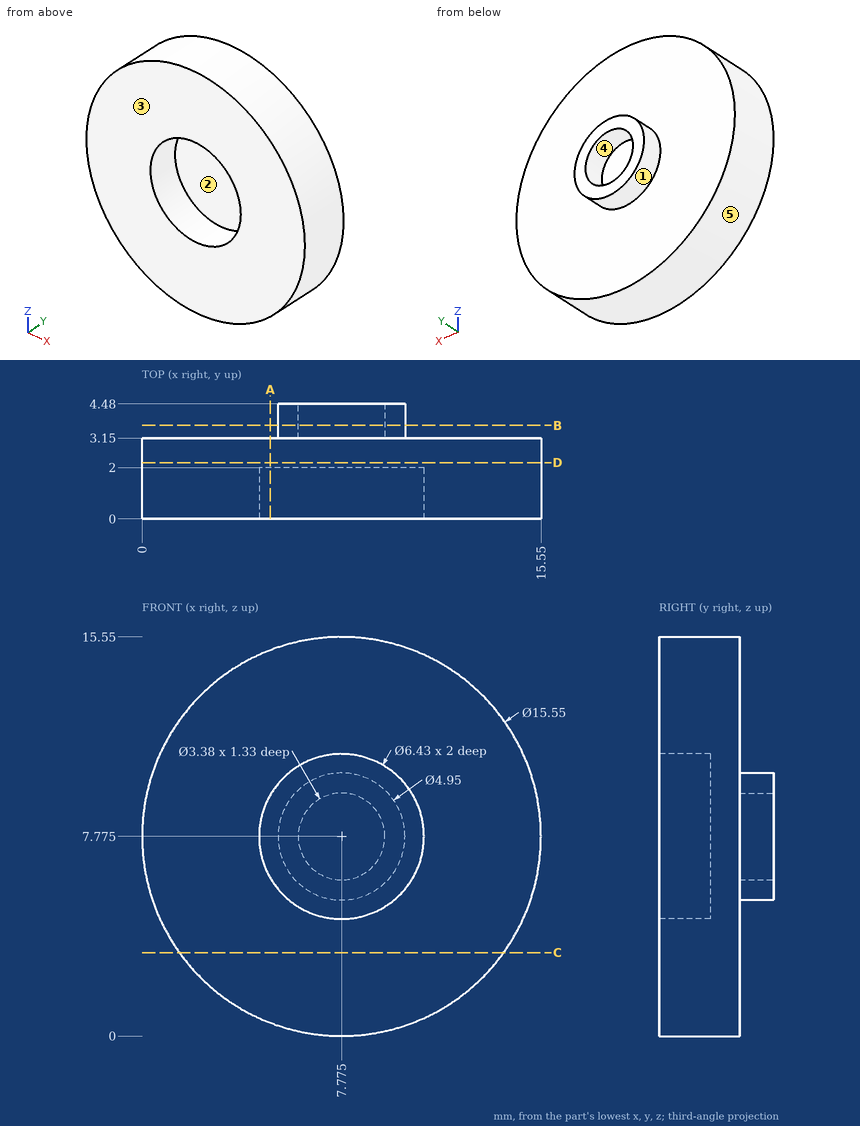
Geometry check sheet. Reference: drawing and pictorial views, mm from the part's lowest x, y, z. A direction names the side the tool comes from. Coordinates: 2 decimals unless noted, no trailing zeros. Order: outer loops, then holes, each group sorted by start corner. A loop starts at its lowest first (then second) coordinate and runs counter-clockwise, first axis right, second up. Notation, with made-up numbers: (36.25, -25) -> (56.25, -25) arc R11 cw to (56.25, -6) -> close; hole circle Ø8 at (18.5, 34). An arc over 180 degrees is marked (long way). Put each result on its own line as item: value. Start each with the question number.
1) Cross-section at D-D (y = 2.2). Enter the section's corners in (x, z) (3 decimals).
2) Cross-section at A-A (x = 5). Enter the section's corners in (y, z), plus the area to 3 significant figures.
3) Tool access check on the marked faces 1 and 2. Record the directions out of +Z, -Z, +X, -X, +Y, -Y that give a thin tool (end or side, any length) a straight path to the whole face; none if there is none.
4) Release check for a two-part mould opening along Z. For the marked faces 3, 4 and 5 record: pulls with the +Z half, pulls with the -Z half, needs draft (parallel to the pull), parting line crosses it, or undercut.
5) Cross-section at C-C (z = 3.25). Enter the section's corners in (x, y).
6) Cross-section at B-B (y = 3.65). Enter the section's corners in (x, z) (3 decimals), plus the area to 3 significant figures.
7) Go/stop test with flat-tipped pins: pin 1 (4 mm diameter, centred on x = 7.775, z = 7.775, fed in from -Y); pin 2 (2 mm diameter, centred on y = 0.5, z = 1.5, fed in from -X); pin 3 (1 mm diameter, centred on y = 3, z = 9, fed in from -X). Record where each tip stops, or that it passes through.
8) Material ranges on L1, parallel to Y at x = 4, z = 6.75; L2, parallel to X at y = 1.85, z = 7.25; L3, parallel to Z at x = 6.5, y = 0.65, recorded low to high.
Geometry check:
1. outline: circle Ø15.55 at (7.775, 7.775)
2. outline: (0, 0.51) -> (3.15, 0.51) -> (3.15, 15.04) -> (0, 15.04) -> (0, 9.4) -> (2, 9.4) -> (2, 6.15) -> (0, 6.15) -> close
2. area: 39.3 mm^2
3. face 1: +Y
3. face 2: -Y
4. face 3: needs draft
4. face 4: undercut
4. face 5: parting line crosses it
5. outline: (1.45, 0) -> (14.1, 0) -> (14.1, 3.15) -> (1.45, 3.15) -> close
6. outline: circle Ø4.95 at (7.775, 7.775); hole circle Ø3.38 at (7.775, 7.775)
6. area: 10.3 mm^2
7. pin 1: stops at y = 2
7. pin 2: stops at x = 2.06
7. pin 3: stops at x = 0.03
8. L1: y = 0 to 3.15
8. L2: x = 0.02 to 4.6, 10.95 to 15.53
8. L3: z = 0.11 to 4.82, 10.73 to 15.44
